Source: three-view drawing plus pictorial views. Frame: mm from the lowest corner of the part. Coordinates: 2 decimals unless noted, no trailing zeros. Write each loop counter-clockwise with the first axis right and the second up, starting at its lowest first coordinate (ties: lowest second). Pieces come first, ordered by that corner, then holes. Notation, with made-up numbers: (5, 56.5) - (63, 56.5) arc R21 ccw to (63, 60.5) - close; hole circle Ø9 at (64, -4.5). An arc over 180 degrees is marked (long way). Put each result on its own line as item: value.
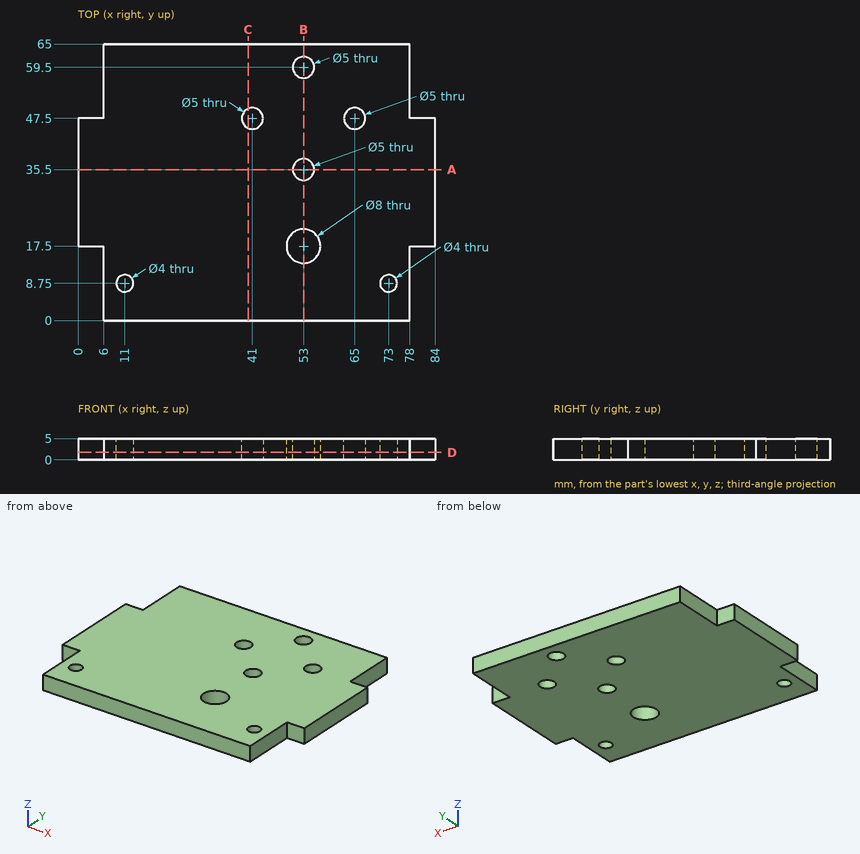
1. Section query A-A (y = 35.5). Return loops of the section in (x, z), then the cut area to 3 significant figures.
Answer below:
outline: (0, 0) - (50.5, 0) - (50.5, 5) - (0, 5) - close; (55.5, 0) - (84, 0) - (84, 5) - (55.5, 5) - close
area: 395 mm²
2. Section query B-B (x = 53). Return loops of the section in (y, z).
Answer below:
outline: (0, 0) - (13.5, 0) - (13.5, 5) - (0, 5) - close; (21.5, 0) - (33, 0) - (33, 5) - (21.5, 5) - close; (38, 0) - (57, 0) - (57, 5) - (38, 5) - close; (62, 0) - (65, 0) - (65, 5) - (62, 5) - close
3. Pin query (flat end, axial travel): pin 1 Ø2.5 at (y, z) = (10, 2.5) entering from +X. Return the tip coordinate at first contact, or that it passes through.
Answer below:
pin 1: stops at x = 78
4. Section query D-D (z = 1.75). Return loops of the section in (x, y), then the cut area to 3 significant figures.
Answer below:
outline: (0, 17.5) - (6, 17.5) - (6, 0) - (78, 0) - (78, 17.5) - (84, 17.5) - (84, 47.5) - (78, 47.5) - (78, 65) - (6, 65) - (6, 47.5) - (0, 47.5) - close; hole circle Ø4 at (11, 8.75); hole circle Ø5 at (41, 47.5); hole circle Ø8 at (53, 17.5); hole circle Ø5 at (53, 35.5); hole circle Ø5 at (53, 59.5); hole circle Ø5 at (65, 47.5); hole circle Ø4 at (73, 8.75)
area: 4,890 mm²
5. Ray query, probe 1 along X at (y, z) = (9, 0.35); probe 2 along Y at (x, z) = (53, 3.4); probe 3 along Y at (x, z) = (65, 1.45). Return the intervals inside material, ascending. Write a range as from..to.
Answer below:
probe 1: x = 6..9.02, 12.98..71.02, 74.98..78
probe 2: y = 0..13.5, 21.5..33, 38..57, 62..65
probe 3: y = 0..45, 50..65
6. Section query C-C (x = 40). Return loops of the section in (y, z).
Answer below:
outline: (0, 0) - (45.21, 0) - (45.21, 5) - (0, 5) - close; (49.79, 0) - (65, 0) - (65, 5) - (49.79, 5) - close
